Input: part model. Units: mm. Frame: model coordinates. A direction names the side the tool comes from. Coordinates: 2 decimals unless noted, no trailing zeros. Order: outer loops, then holes, each group sorted by start corner. A loop starts at its lowest first (then second) coordinate and runs counter-clockwise, first axis right, second up.
Autodesk Inventor part; units mm, degrees
ref_plane "YZ Plane" through (0, 0, 0) normal (1, 0, 0) x (0, 1, 0)
ref_plane "XZ Plane" through (0, 0, 0) normal (0, 1, 0) x (-1, 0, 0)
ref_plane "XY Plane" through (0, 0, 0) normal (0, 0, 1) x (1, 0, 0)
sketch "Szkic1" plane through (0, 0, 0) normal (0, 1, 0) x (-1, 0, 0)
  line L0 (0, 0) -> (12, 0)
  line L1 (12, 0) -> (12, 26)
  line L2 (12, 26) -> (0, 26)
  line L3 (0, 26) -> (0, 0)
  dimension "d0" = 26
  dimension "d1" = 12
extrude "Wyciągnięcie proste1" add sketch "Szkic1" along normal blind 10
fillet "Zaokrąglenie1" radius 2.9 4 edges at (0, 10, 13) (0, 0, 13) (-12, 10, 13) (-12, 0, 13)
sketch "Szkic2" plane through (-9.1, 0, 26) normal (0, 0, 1) x (1, 0, 0)
  circle A0 centre (3.1, 5) radius 2
  line L0 (-2.9, 2.9) -> (-2.9, 7.1)
  line L1 (0, 10) -> (6.2, 10)
  point P0 (9.1, 0)
  point P1 (-2.9, 5)
  point P2 (3.1, 10)
  dimension "d5" = 4
extrude "Wyciągnięcie proste2" add sketch "Szkic2" along normal blind 0.7
sketch "Szkic3" plane through (-6, 5, 26.7) normal (0, 0, 1) x (1, 0, 0)
  circle A0 centre (0, 0) radius 1.5
  line L0 (-1.118, 1) -> (1.118, 1)
  circle A1 centre (0, 0) radius 2
  line L1 (-3.1, -5) -> (3.1, -5)
  point P0 (6, -5)
  dimension "d8" = 3
  dimension "d9" = 2.5
  dimension "d10" = 0
  dimension "d11" = 0
extrude "Wyciągnięcie proste3" add sketch "Szkic3" along normal blind 10 contours A0 L0 picked at (0.0594, 0.1702)
sketch "Szkic4" plane through (0, 10, 0) normal (0, 1, 0) x (1, 0, 0)
  line L0 (-9.1, -26) -> (-12, -26)
  line L1 (0, 0) -> (0, -26)
  line L2 (-12, -26) -> (0, -26)
  line L3 (0, -26) -> (0, -15.4)
  line L4 (0, -15.4) -> (-12, -15.4)
  line L5 (-12, -15.4) -> (-12, -26)
  line L6 (-2.9, 0) -> (-9.1, 0)
  dimension "d14" = 15.4
extrude "Wyciągnięcie proste4" add sketch "Szkic4" against normal blind 10
properties part number "Silniczek"
Item 1: Cut plane A-A on x = -6. Return loops of the section in (y, z), then the cut area to 3 significant figures.
Response values:
outline: (0, 0) - (10, 0) - (10, 26) - (7, 26) - (7, 26.7) - (6, 26.7) - (6, 36.7) - (3.5, 36.7) - (3.5, 26.7) - (3, 26.7) - (3, 26) - (0, 26) - close
area: 288 mm2
Item 2: Cut plane B-B on z = 4. Return loops of the section in (x, y).
Response values:
outline: (-12, 2.9) arc R2.9 ccw to (-9.1, 0) - (-2.9, 0) arc R2.9 ccw to (0, 2.9) - (0, 7.1) arc R2.9 ccw to (-2.9, 10) - (-9.1, 10) arc R2.9 ccw to (-12, 7.1) - close
Item 3: Pin query (flat end, axial travel): pin 1 Ø1.8 at (x, z) = (-5.5, 33) entering from +Y. Return the tip coordinate at first contact, or that it passes through.
Response values:
pin 1: stops at y = 6
Item 4: Cut plane C-C on y = 5. Return loops of the section in (x, z).
Response values:
outline: (-12, 0) - (0, 0) - (0, 26) - (-4, 26) - (-4, 26.7) - (-4.5, 26.7) - (-4.5, 36.7) - (-7.5, 36.7) - (-7.5, 26.7) - (-8, 26.7) - (-8, 26) - (-12, 26) - close
Item 5: Access query for faces 1 (the face through (-11.2, 0.9, 7.8)), 2 (the face through (-11.3, 9.4, 15.4)), 3 (the face through (-6, 6.4, 26.7)). Directions: +Z, -Z, +X, -X, +Y, -Y. A direction counts if a zero-diameter tool reaches every point of the face in a straight line with its end or side. Return the directions, or none.
Response values:
face 1: -Z, -X, -Y
face 2: -Z, -X, +Y
face 3: +Z
Item 6: Cut plane D-D on y = 1. Return loops of the section in (x, z).
Response values:
outline: (-12, 15.4) - (-11.29, 15.4) - (-11.29, 0) - (-0.71, 0) - (-0.71, 15.4) - (0, 15.4) - (0, 26) - (-12, 26) - close
Item 7: Ray query, probe 1 along Y at (x, z) = (-2.75, 11.5); probe 2 along Z at (x, y) = (-9.75, 7.5); probe 3 along X at (y, z) = (4.25, 33.5). Return the intervals inside material, ascending.
Response values:
probe 1: y = 0 to 10
probe 2: z = 0 to 26
probe 3: x = -7.3 to -4.7
